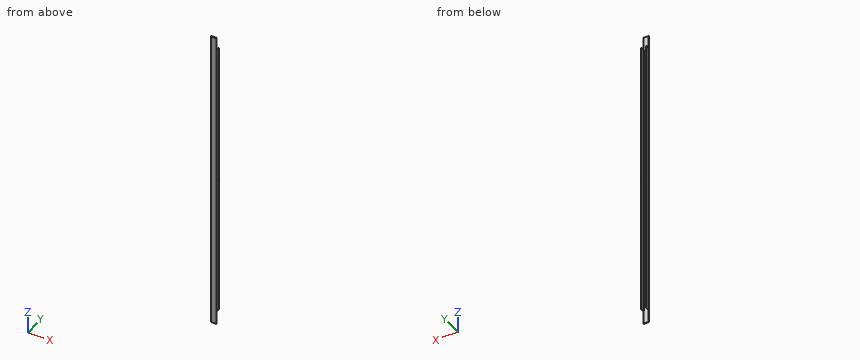
```python
from build123d import *

# Parameters (mm, degrees)
F1_DEPTH = 903.3002
F2_W     = 1.5875
F2_H     = 38.9001
F2_H_2   = 0.635
F3_DEPTH = 11.1125
F4_W     = 1.5875
F4_H     = 38.1127
F5_DEPTH = 11.1125


with BuildPart() as f1:
    # F0 (on Top) → F1 (new body)
    with BuildSketch(Plane.XY):
        Polygon((-6.35, -6.35), (6.35, -6.35), (7.9375, -6.35), (7.9375, 6.35), (6.35, 6.35), (6.35, -4.7625), (-6.35, -4.7625), (-6.35, 6.35), (-7.9375, 6.35), (-7.9375, -6.35), align=None)
    extrude(amount=F1_DEPTH)

    # F2 (on face) → F3 (cut)
    with BuildSketch(Plane(origin=(0, 6.35, 0), x_dir=(-1, 0, 0), z_dir=(0, 1, 0))):
        with Locations((-7.14375, 19.45005)):
            Rectangle(F2_W, F2_H)
        with Locations((-7.14375, 883.85015)):
            Rectangle(F2_W, F2_H)
        with Locations((-7.14375, 451.6501)):
            Rectangle(F2_W, F2_H_2)
    extrude(amount=-F3_DEPTH, mode=Mode.SUBTRACT)

    # F4 (on face) → F5 (cut)
    with BuildSketch(Plane(origin=(0, 6.35, 0), x_dir=(-1, 0, 0), z_dir=(0, 1, 0))):
        with Locations((7.14375, 19.05635)):
            Rectangle(F4_W, F4_H)
        with Locations((7.14375, 884.24385)):
            Rectangle(F4_W, F4_H)
    extrude(amount=-F5_DEPTH, mode=Mode.SUBTRACT)


solid = f1.part
```
CAD build for the part. Positions are in the model's coordinates, mm. Round coordinates to 2 decimals unless told otherwise and drop trailing zeros. Loops run counter-clockwise (first coordinate to the right, second up) from the corner with the lowest first, then second, coordinate; pieces in that order, holes last. Notation, with made-up numbers: (16, -19.75) - (43, -19.75) arc R23 ccw to (43, 9.25) - close; hole circle Ø1 at (29.25, -20). An arc over 180 degrees is marked (long way). Return JSON: item names as keys, results as strings. Group by question number.
Q1. Flat gauge pins, fed straight in: pin 1 Ø1.3 at (x, y) = (7.5, 2) entering from -Z; pin 2 Ø2 at (x, z) = (-4, 96) entering from +Y; pin 3 Ø0.8 at (x, y) = (-7, 2.5) entering from +Z. Where does each tip first touch, or does it go through?
Q2. Band-saw the part on B-B on z = 707.5. Give the cut face in (x, y), plus the area to 3 significant figures.
Q3. Band-saw the part on A-A on y = 1. Give the cut face in (x, z), plus the area to 3 significant figures.
Q4. Band-saw the part on C-C on x = -2. Give the cut face in (y, z), plus the area to 3 significant figures.
Q5. Drill centre lines: line 1 along X through (y, z) = (-4.25, 458); line 2 along Y through (x, z) = (-6.25, 61); line 3 along Z through (x, y) = (-6.5, -2.75). Where is each one in solid material? Low to high. Write a range as [from, to].
Solutions:
{
 "1": {"pin 1": "stops at z = 38.9", "pin 2": "stops at y = -4.76", "pin 3": "stops at z = 865.19"},
 "2": {"outline": "(-7.94, -6.35) - (7.94, -6.35) - (7.94, 6.35) - (6.35, 6.35) - (6.35, -4.76) - (-6.35, -4.76) - (-6.35, 6.35) - (-7.94, 6.35) - close", "area": "60.5 mm^2"},
 "3": {"outline": "(-7.94, 38.11) - (-6.35, 38.11) - (-6.35, 865.19) - (-7.94, 865.19) - close; (6.35, 38.9) - (7.94, 38.9) - (7.94, 451.33) - (6.35, 451.33) - close; (6.35, 451.97) - (7.94, 451.97) - (7.94, 864.4) - (6.35, 864.4) - close", "area": "2,620 mm^2"},
 "4": {"outline": "(-6.35, 0) - (-4.76, 0) - (-4.76, 903.3) - (-6.35, 903.3) - close", "area": "1,430 mm^2"},
 "5": {"line 1": "x = [-7.94, -6.35], [6.35, 7.94]", "line 2": "y = [-6.35, -4.76]", "line 3": "z = [38.11, 865.19]"}
}
